Check sheet for the modelled part. Datum: model origin and axes. Units: mm. A direction names the side the tool comes from. Coordinates: 2 decimals unless noted, no trailing zeros. Loops run counter-clockwise (first coordinate to the right, second up) from the corner with the lowest first, then second, coordinate; pieces in that order, holes last. Notation, with made-up numbers: (17, 75.5) - (63, 75.5) arc R31 cw to (63, 104.5) - close; hole circle Ø3 at (62, 8). An arc over 180 degrees is marked (long way). Use a Markdown table: item, result. Add a question column.
1) Sectioned sample at B-B, the plane y = 47. Enter the section's corners in (x, z).
2) Draft check along Y on faces 6 (the flat face through (-7, 29, 0)), 7 (the flat face through (12, 66, 99)), 8 (the flat face through (2.909, 12.884, 107.605)). Enter one of: pulls with the +Y half, pulls with the -Y half, needs draft (parallel to the pull), parting line crosses it, or undercut.
3) Sectioned sample at D-D, the plane x = -28.5. Enter the section's corners in (y, z).
4) Go/stop test with flat-tipped pins: P1, Ø4.5, axis at y = 75, z = 89, coming from the +X side; P2, Ø10, axis at x = 8.5, z = 14, coming from the -Y side; P3, Ø4.5, axis at y = 62, z = 16, coming from the +X side. Record where each tip stops, or that it passes through.
5) Tool access check on faces 1 (the flat face through (15, 58, 13)), 2 (the flat face through (-5, 58, -5)), 3 (the flat face through (12, 51, 99)), 4 (the flat face through (-4, 56, 37)), 5 (the cylindrical face through (30, 8, 95)). Record the directions out of +Z, -Z, +X, -X, +Y, -Y that give a thin tool (end or side, any length) a straight path to the whole face; none if there is none.
6) Sectioned sample at A-A, the plane z = 45. Enter the section's corners in (x, y).
7) Sectioned sample at C-C, the plane x = 26.5. Enter the section's corners in (y, z), then the cut area to 3 significant figures.
8) Thickness scan on line 1 (Z direction, x = 29.5, y = 3.5); line 2 (Z direction, x = -12.5, y = 66.5); line 3 (Z direction, x = 4, y = 18). Record the ranges inside material, lowest first.
from build123d import *

# Parameters (mm, degrees)
BOSS_EXTRUDE1_DEPTH      = 115
CUT_EXTRUDE1_DEPTH       = 1
CUT_EXTRUDE1_DEPTH_BACK  = 15
SKETCH3_W                = 20
SKETCH3_H                = 15
BOSS_EXTRUDE2_DEPTH      = 10
BOSS_EXTRUDE2_DEPTH_BACK = 110
SKETCH4_W                = 33
SKETCH4_H                = 40
CUT_EXTRUDE2_DEPTH       = 31
CUT_EXTRUDE2_DEPTH_BACK  = 46.5
CUT_EXTRUDE4_DEPTH       = 67
CUT_EXTRUDE4_DEPTH_BACK  = 41.362796982
FILLET1_R                = 10


with BuildPart() as part:
    # Sketch1 → Boss-Extrude1 (new body)
    with BuildSketch(Plane.XY):
        with BuildLine():
            Line((0, 0), (40, 0))
            Line((40, 0), (40, 15))
            Line((40, 15), (10, 15))
            Line((10, 15), (10, 81))
            ThreePointArc((10, 81), (-35.256322222, 31.603413808), (0, -25.362796982))
            Line((0, -25.362796982), (0, 0))
        make_face()
    extrude(amount=BOSS_EXTRUDE1_DEPTH)

    # Sketch2 → Cut-Extrude1 (cut, two sides)
    with BuildSketch(Plane.XY.offset(115)) as cut_extrude1_sk:
        with BuildLine():
            Line((40, 5), (-35.235044142, 20.9917023))
            ThreePointArc((-35.235044142, 20.9917023), (-24.318751046, 59.816391467), (10, 81))
            Line((10, 81), (10, 15))
            Line((10, 15), (40, 15))
            Line((40, 15), (40, 5))
        make_face()
    extrude(amount=CUT_EXTRUDE1_DEPTH, mode=Mode.SUBTRACT)
    extrude(cut_extrude1_sk.sketch, amount=-CUT_EXTRUDE1_DEPTH_BACK, mode=Mode.SUBTRACT)

    # Sketch3 → Boss-Extrude2 (add, two sides)
    with BuildSketch(Plane(origin=(0, 0, 0), x_dir=(-1, 0, 0), z_dir=(0, 0, -1))) as boss_extrude2_sk:
        with Locations((-5, 58.5)):
            Rectangle(SKETCH3_W, SKETCH3_H)
    extrude(amount=BOSS_EXTRUDE2_DEPTH)
    extrude(boss_extrude2_sk.sketch, amount=-BOSS_EXTRUDE2_DEPTH_BACK)

    # Sketch4 → Cut-Extrude2 (cut, two sides)
    with BuildSketch(Plane(origin=(10, 0, 0), x_dir=(0, 0, -1), z_dir=(1, 0, 0))) as cut_extrude2_sk:
        with Locations((-53.5, 61)):
            Rectangle(SKETCH4_W, SKETCH4_H)
    extrude(amount=CUT_EXTRUDE2_DEPTH, mode=Mode.SUBTRACT)
    extrude(cut_extrude2_sk.sketch, amount=-CUT_EXTRUDE2_DEPTH_BACK, mode=Mode.SUBTRACT)

    # Sketch6 → Cut-Extrude4 (cut, two sides)
    with BuildSketch(Plane(origin=(0, 15, 0), x_dir=(1, 0, 0), z_dir=(0, 1, 0))) as cut_extrude4_sk:
        with BuildLine():
            Line((35, -10), (35, -90))
            ThreePointArc((35, -90), (30, -95), (25, -90))
            Line((25, -90), (25, -10))
            ThreePointArc((25, -10), (30, -5), (35, -10))
        make_face()
    extrude(amount=CUT_EXTRUDE4_DEPTH, mode=Mode.SUBTRACT)
    extrude(cut_extrude4_sk.sketch, amount=-CUT_EXTRUDE4_DEPTH_BACK, mode=Mode.SUBTRACT)

    # Fillet1
    fillet1_edges = [part.edges().sort_by_distance(p)[0] for p in [
        (10, 15, 50),
    ]]
    fillet(fillet1_edges, radius=FILLET1_R)


solid = part.part
Solved:
| question | item | result |
|---|---|---|
| 1 | outline | (-31.54, 0) - (10, 0) - (10, 37) - (-31.54, 37) - close; (-31.54, 70) - (10, 70) - (10, 100) - (-31.54, 100) - close |
| 2 | face 6 | needs draft |
| 2 | face 7 | pulls with the +Y half |
| 2 | face 8 | undercut |
| 3 | outline | (-0.57, 0) - (53.39, 0) - (53.39, 37) - (41, 37) - (41, 70) - (53.39, 70) - (53.39, 100) - (19.56, 100) - (19.56, 115) - (-0.57, 115) - close |
| 4 | P1 | stops at x = 10 |
| 4 | P2 | stops at y = 0 |
| 4 | P3 | stops at x = 15 |
| 5 | face 1 | +Z, -Z, +X, +Y |
| 5 | face 2 | -Z, -X, +Y, -Y |
| 5 | face 3 | +Z, +X |
| 5 | face 4 | +X, -X, +Y |
| 5 | face 5 | +Y, -Y |
| 6 | outline | (-33.55, 41) arc R55.5 ccw to (0, -25.36) - (0, 0) - (25, 0) - (25, 15) - (20, 15) arc R10 cw to (10, 25) - (10, 41) - close; (35, 0) - (40, 0) - (40, 15) - (35, 15) - close |
| 7 | outline | (0, 0) - (15, 0) - (15, 6.43) - (0, 6.43) - close; (0, 93.57) - (15, 93.57) - (15, 100) - (7.87, 100) - (7.87, 115) - (0, 115) - close |
| 7 | area | 311 mm2 |
| 8 | line 1 | z = 0 to 5.03, 94.97 to 115 |
| 8 | line 2 | z = 0 to 37, 70 to 100 |
| 8 | line 3 | z = 0 to 100 |
